from build123d import *

# Parameters (mm, degrees)
ESBO_O1_R                = 1.6
RESSALTO_EXTRUS_O1_DEPTH = 3


with BuildPart() as part:
    # Esboço1 → Ressalto-extrusão1 (new body)
    with BuildSketch(Plane.XZ.offset(3)):
        with BuildLine():
            Line((-7.1, -33.6), (7.1, -33.6))
            ThreePointArc((7.1, -33.6), (14.171067812, -30.671067812), (17.1, -23.6))
            Line((17.1, -23.6), (17.1, -6))
            Line((17.1, -6), (7.5, -6))
            Line((7.5, -6), (7.5, 0))
            Line((7.5, 0), (-7.5, 0))
            Line((-7.5, 0), (-7.5, -6))
            Line((-7.5, -6), (-17.1, -6))
            Line((-17.1, -6), (-17.1, -23.6))
            ThreePointArc((-17.1, -23.6), (-14.171067812, -30.671067812), (-7.1, -33.6))
        make_face()
        with Locations((-12.5, -27)):
            Circle(ESBO_O1_R, mode=Mode.SUBTRACT)
        with Locations((12.5, -27)):
            Circle(ESBO_O1_R, mode=Mode.SUBTRACT)
    extrude(amount=-RESSALTO_EXTRUS_O1_DEPTH)


solid = part.part
Part model, mm, in its own coordinate system. A direction names the side the tool comes from. Give positions to 0.01 mm unless a question says otherwise; leave off trailing zeros. Order: outer loops, then holes, each group sorted by start corner. A loop starts at its lowest first (then second) coordinate and runs counter-clockwise, first axis right, second up. Notation, with made-up numbers: (60.25, 24.5) - (101.25, 24.5) arc R18 ccw to (101.25, 30.5) - close; hole circle Ø11 at (24, 81.5). An arc over 180 degrees is marked (long way). Use a Markdown table: item, result.
1) Saw through at D-D on x = 9. List the corners of the cut face in (y, z).
Checked values:
| item | result |
|---|---|
| outline | (-3, -33.42) - (0, -33.42) - (0, -6) - (-3, -6) - close |
2) Saw through at B-B on z = -27. List the corners of the cut face in (x, y), plus the area to 3 significant figures.
Checked values:
| item | result |
|---|---|
| outline | (-16.5, -3) - (-14.1, -3) - (-14.1, 0) - (-16.5, 0) - close; (-10.9, -3) - (10.9, -3) - (10.9, 0) - (-10.9, 0) - close; (14.1, -3) - (16.5, -3) - (16.5, 0) - (14.1, 0) - close |
| area | 79.8 mm² |
3) Flat gauge pins, fed straight in: P1, Ø1, axis at y = -1, z = -27, coming from the +X side; P2, Ø0.9, axis at y = -1.5, z = -2, coming from the +X side; P3, Ø0.9, axis at x = 11.5, y = -2, coming from the +Z side. Where does each tip first touch, or does it go through?
Checked values:
| item | result |
|---|---|
| P1 | x = 16.67 |
| P2 | x = 7.5 |
| P3 | z = -6 |
4) Saw through at A-A on y = -2.25. List the corners of the cut face in (x, z).
Checked values:
| item | result |
|---|---|
| outline | (-17.1, -23.6) arc R10 ccw to (-7.1, -33.6) - (7.1, -33.6) arc R10 ccw to (17.1, -23.6) - (17.1, -6) - (7.5, -6) - (7.5, 0) - (-7.5, 0) - (-7.5, -6) - (-17.1, -6) - close; hole circle Ø3.2 at (-12.5, -27); hole circle Ø3.2 at (12.5, -27) |
5) Probe L1, parallel to X at y = -0.15, z = -26; L2, parallel to Z at x = 12.5, y = -1.85; L3, parallel to Z at x = 12, y = -2.35. List the from-to ranges inside material, lowest first. Write a range as from..to.
Checked values:
| item | result |
|---|---|
| L1 | -16.81..-13.75, -11.25..11.25, 13.75..16.81 |
| L2 | -32.02..-28.6, -25.4..-6 |
| L3 | -32.32..-28.52, -25.48..-6 |
6) Two-plate mould, pull along X, no slides. Class faces 1 (the flat face through (-7.5, -2, -3)), 2 (the cylindrical face through (-13.68, -1.52, -25.92)), 3 (the flat face through (0, -3, -17)), 4 (the cylindrical face through (14.09, -1.52, -30.75)): +X half, -X half, draft (parallel to the pull), parting line (faces both ways), or undercut.
Checked values:
| item | result |
|---|---|
| face 1 | -X half |
| face 2 | undercut |
| face 3 | draft |
| face 4 | +X half |
7) 3-axis set-ups, long thin cutter, end or side, ignore diameter. For faces 5 (the flat face through (7.5, -2, -3)), 6 (the flat face through (-12, -2, -6)), 7 (the flat face through (0, 0, -17)): which of +Z, -Z, +X, -X, +Y, -Y reach the whole face in a straight line?
Checked values:
| item | result |
|---|---|
| face 5 | +Z, +X, +Y, -Y |
| face 6 | +Z, -X, +Y, -Y |
| face 7 | +Z, -Z, +X, -X, +Y |
8) Saw through at C-C on x = 12.5. List the corners of the cut face in (y, z).
Checked values:
| item | result |
|---|---|
| outline | (-3, -32.02) - (0, -32.02) - (0, -28.6) - (-3, -28.6) - close; (-3, -25.4) - (0, -25.4) - (0, -6) - (-3, -6) - close |
